Read the model definition and answer for the solid it produces. Units are mm, in the model's axes. Face numbers are marked on the shaded views. A direction names the side the tool comes from. Coordinates: 2 decimals unless noted, no trailing zeros. Write each loop counter-clockwise with the first axis right and the second up, starting at its lowest first coordinate (ties: lowest second). Pieces come first, ordered by that corner, then holes. Notation, with made-up numbers: (-30, 54) - (8, 54) arc R5 ccw to (8, 62) - close; hole circle Ø10 at (-28, 26.5). An arc over 180 degrees is marked (long way). Use a Markdown table: item, result.
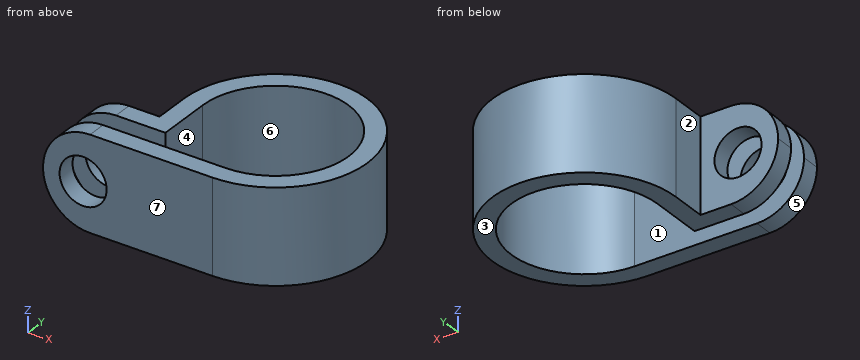
from build123d import *

# Parameters (mm, degrees)
F1_DEPTH = 10
F2_R     = 4.99999
F4_D     = 5


# Not quite as in the source:
# - a fillet or chamfer is up to 0.001 mm smaller than in the source, because OpenCascade refuses the exact size


with BuildPart() as f1:
    # F0 (on Top) → F1 (new body)
    with BuildSketch(Plane.XY):
        with BuildLine():
            ThreePointArc((-7.75, 0), (5.4800775542, 5.4800775542), (0, -7.75))
            Line((0, -7.75), (-18, -7.75))
            Line((-18, -7.75), (-18, -9.75))
            Line((-18, -9.75), (0, -9.75))
            ThreePointArc((0, -9.75), (6.8942911166, 6.8942911166), (-9.75, 0))
            Line((-9.75, 0), (-9.75, -3.75))
            Line((-9.75, -3.75), (-18, -3.75))
            Line((-18, -3.75), (-18, -5.75))
            Line((-18, -5.75), (-7.75, -5.75))
            Line((-7.75, -5.75), (-7.75, 0))
        make_face()
    extrude(amount=F1_DEPTH)

    # F2 (radius 5 in the source; OpenCascade refuses exactly that, so slightly less here)
    f2_edges = [f1.edges().sort_by_distance(p)[0] for p in [
        (-18, -4.75, 0),
        (-18, -8.75, 0),
        (-18, -8.75, 10),
        (-18, -4.75, 10),
    ]]
    fillet(f2_edges, radius=F2_R)

    # F4 (through all)
    with Locations(Plane(origin=(0, -3.75, 0), x_dir=(-1, 0, 0), z_dir=(0, 1, 0))):
        with Locations((13.740055263, 5)):
            Hole(F4_D / 2)


solid = f1.part
(1) For the marked faces 1, 2 and 3, determine the directions among +Z, -Z, +X, -X, +Y, -Y from which every point of the face is accessible in a straight line to the end or side of a thin tool.
Report:
| item | result |
|---|---|
| face 1 | +Z, -Z, -X |
| face 2 | +Z, -Z, -X, +Y |
| face 3 | -Z, +X, -X, +Y, -Y |
(2) Each of these flat-tipped pins is pushed along its axis until it touches: P1, Ø3, axis at y = -6.5, z = 1.5, coming from the -X side; P2, Ø1.5, axis at y = 5.5, z = 4.5, coming from the +X side; P3, Ø3, axis at y = -1.5, z = 6, coming from the -X side. Where does it stop, or does it pass through?
Report:
| item | result |
|---|---|
| P1 | stops at x = -17.49 |
| P2 | stops at x = 8.51 |
| P3 | stops at x = -9.75 |
(3) A cutting plane is placed at A-A, the plane y = -4.75. Count the separate pieces of the cut face and the enclosed holes in it, and give its area (3 significant figures).
Report:
| item | result |
|---|---|
| separate pieces | 2 |
| enclosed holes | 1 |
| area | 96.0 mm² |
(4) A cutting plane is placed at B-B, the plane y = 1.25. Write down the section's boundary in (x, z).
Report:
| item | result |
|---|---|
| outline | (-9.67, 0) - (-7.65, 0) - (-7.65, 10) - (-9.67, 10) - close; (7.65, 0) - (9.67, 0) - (9.67, 10) - (7.65, 10) - close |
(5) A cutting plane is placed at D-D, the plane x = -2.5. Write down the section's boundary in (y, z), and give its area (3 significant figures).
Report:
| item | result |
|---|---|
| outline | (-9.75, 0) - (-7.75, 0) - (-7.75, 10) - (-9.75, 10) - close; (7.34, 0) - (9.42, 0) - (9.42, 10) - (7.34, 10) - close |
| area | 40.9 mm² |
(6) The mould has two halves that part along Y. Classify the marked faces 4, 5, 6 and 7: pulls with the +Y half, pulls with the -Y half, needs draft (parallel to the pull), parting line crosses it, or undercut.
Report:
| item | result |
|---|---|
| face 4 | undercut |
| face 5 | needs draft |
| face 6 | undercut |
| face 7 | pulls with the -Y half |
(7) A cutting plane is placed at C-C, the plane z = 6.75. Write down the section's boundary in (x, y).
Report:
| item | result |
|---|---|
| outline | (-17.68, -9.75) - (-15.53, -9.75) - (-15.53, -7.75) - (-17.68, -7.75) - close; (-17.68, -5.75) - (-15.53, -5.75) - (-15.53, -3.75) - (-17.68, -3.75) - close; (-11.95, -9.75) - (0, -9.75) arc R9.75 ccw (long way) to (-9.75, 0) - (-9.75, -3.75) - (-11.95, -3.75) - (-11.95, -5.75) - (-7.75, -5.75) - (-7.75, 0) arc R7.75 cw (long way) to (0, -7.75) - (-11.95, -7.75) - close |
(8) Straight lines are drawn through the part: L1, parallel to Y at x = -13.5, z = 9; L2, parallel to X at y = -4, z = 6.25 (3 decimals); L3, parallel to Y at x = 5.5, z = 7.25. For each, find the intervals that lie inside material, in ascending order.
Report:
| item | result |
|---|---|
| L1 | y = -9.75 to -7.75, -5.75 to -3.75 |
| L2 | x = -17.841 to -15.905, -11.575 to -7.75, 6.638 to 8.892 |
| L3 | y = -8.05 to -5.46, 5.46 to 8.05 |
